Read the model definition and answer for the solid it produces. Units are mm, in the model's axes. Give positions to 0.01 mm unless a question says otherwise; leave off trailing zeros. Write each loop counter-clockwise with the first axis right and the second up, starting at its lowest first coordinate (ties: lowest second). Pieces come first, ordered by that corner, then holes. Notation, with made-up numbers: M -14.5,45.5 L 31.5,45.5 A13 ccw 31.5,52.5 Z; hole C 9.25,55 d4. An arc over 180 degrees is marked long. Put each result on its own line as item: value.
Autodesk Inventor part; units mm, degrees
ref_plane "YZ Plane" through (0, 0, 0) normal (1, 0, 0) x (0, 1, 0)
ref_plane "XZ Plane" through (0, 0, 0) normal (0, 1, 0) x (-1, 0, 0)
ref_plane "XY Plane" through (0, 0, 0) normal (0, 0, 1) x (1, 0, 0)
sketch "スケッチ2" plane through (0, 0, 0) normal (0, 1, 0) x (-1, 0, 0)
  circle A0 centre (366.8992, 83.5559) radius 3
  circle A1 centre (432.0925, 120.7557) radius 3
  arc A2 (460.0993, 143.4366) -> (457.2735, 146.2345) centre (458.5344, 144.682) ccw
  arc A3 (400.439, 89.2207) -> (460.0993, 143.4366) centre (263.302, 300.0629) ccw
  arc A4 (391.277, 83.6402) -> (400.439, 89.2207) centre (301.619, 241.1522) ccw
  arc A5 (372.7132, 76.1699) -> (391.277, 83.6402) centre (354.4726, 148.2986) ccw
  arc A6 (360.1081, 74.8804) -> (372.7132, 76.1699) centre (362.0183, 118.4608) ccw
  arc A7 (355.7086, 75.8282) -> (360.1081, 74.8804) centre (360.696, 88.2936) ccw
  arc A8 (354.3762, 83.2451) -> (355.7086, 75.8282) centre (357.3588, 79.9528) ccw
  arc A9 (361.0987, 88.3442) -> (354.3762, 83.2451) centre (386.9085, 47.3355) ccw
  arc A10 (385.4553, 102.095) -> (361.0987, 88.3442) centre (517.0615, -159.4623) ccw
  arc A11 (385.4553, 102.095) -> (400.8032, 109.8486) centre (-2010.0977, 4863.0707) ccw
  arc A12 (400.8032, 109.8486) -> (428.5996, 125.6368) centre (247.4107, 412.2703) ccw
  arc A13 (428.5996, 125.6368) -> (457.2735, 146.2345) centre (269.2327, 377.7487) ccw
  circle A14 centre (287.1934, 37.1564) radius 3
  circle A15 centre (359.7933, 56.2153) radius 3
  arc A16 (392.7161, 70.8747) -> (390.7107, 74.3087) centre (391.5269, 72.4828) ccw
  arc A17 (321.0565, 33.9474) -> (392.7161, 70.8747) centre (243.1623, 273.099) ccw
  arc A18 (310.7624, 30.9284) -> (321.0565, 33.9474) centre (264.9264, 206.2785) ccw
  arc A19 (290.8977, 28.5173) -> (310.7624, 30.9284) centre (291.9468, 102.9093) ccw
  arc A20 (278.3883, 30.5342) -> (290.8977, 28.5173) centre (291.5128, 72.1352) ccw
  arc A21 (274.384, 32.5883) -> (278.3883, 30.5342) centre (282.4278, 43.3382) ccw
  arc A22 (275.0166, 40.0974) -> (274.384, 32.5883) centre (277.0456, 36.1453) ccw
  arc A23 (282.8299, 43.2828) -> (275.0166, 40.0974) centre (297.1464, -3.0086) ccw
  arc A24 (309.9154, 50.2611) -> (282.8299, 43.2828) centre (369.3413, -236.446) ccw
  arc A25 (309.9154, 50.2611) -> (326.7472, 53.7782) centre (-771.7798, 5269.0252) ccw
  arc A26 (326.7472, 53.7782) -> (357.6827, 61.8342) centre (256.8539, 385.5961) ccw
  arc A27 (357.6827, 61.8342) -> (390.7107, 74.3087) centre (268.9975, 346.6028) ccw
  circle A28 centre (20.0666, -1.5588) radius 5
  circle A29 centre (130.4331, -10.1322) radius 5
  arc A30 (313.248, 18.4984) -> (312.0524, 22.2894) centre (312.4376, 20.3268) ccw
  arc A31 (100.6618, -32.4332) -> (313.248, 18.4984) centre (68.6386, 570.3585) ccw
  arc A32 (74.9225, -33.0376) -> (100.6618, -32.4332) centre (77.5861, 401.9345) ccw
  arc A33 (27.374, -26.2879) -> (74.9225, -33.0376) centre (76.0159, 145.5175) ccw
  arc A34 (-0.3728, -13.8419) -> (27.374, -26.2879) centre (55.8939, 74.446) ccw
  arc A35 (-8.3795, -6.5926) -> (-0.3728, -13.8419) centre (16.9451, 13.3315) ccw
  arc A36 (-2.2486, 10.4222) -> (-8.3795, -6.5926) centre (0, 0) ccw
  arc A37 (17.8428, 12.9532) -> (-2.2486, 10.4222) centre (22.277, -103.2534) ccw
  arc A38 (84.9679, 12.306) -> (17.8428, 12.9532) centre (44.6377, -689.2581) ccw
  arc A39 (84.9679, 12.306) -> (126.1724, 10.004) centre (819.0754, 12782.4716) ccw
  arc A40 (126.1724, 10.004) -> (202.8919, 9.4636) centre (170.258, 822.6468) ccw
  arc A41 (202.8919, 9.4636) -> (312.0524, 22.2894) centre (174.1884, 724.7085) ccw
  line L0 (400.439, 89.2207) -> (374.6007, 72.4148)
  line L1 (374.6007, 72.4148) -> (391.2826, 74.4678)
  line L2 (355.7086, 75.8282) -> (369.1755, 70.4401)
  line L3 (369.1755, 70.4401) -> (326.7472, 53.7782)
  line L4 (321.0565, 33.9474) -> (289.8884, 23.7957)
  line L5 (289.8884, 23.7957) -> (312.5672, 22.3226)
  line L6 (278.3883, 30.5342) -> (291.6044, 26.3646)
  line L7 (291.6044, 26.3646) -> (243.2783, 12.2299)
  point P0 (0, 0)
extrude "押し出し2" add sketch "スケッチ2" along normal blind 4
fillet "フィレット2" radius 3 4 edges at (-369.1755, 2, 70.4401) (-291.6044, 2, 26.3646) (-374.6007, 2, 72.4148) (-289.8884, 2, 23.7957)
fillet "フィレット2" radius 100 2 edges at (-326.7472, 2, 53.7782) (-243.2783, 2, 12.2299)
sketch "スケッチ3" plane through (0, 0, 0) normal (0, -1, 0) x (1, 0, 0)
  circle A0 centre (-20.0666, -1.5588) radius 6
  circle A1 centre (-130.4331, -10.1322) radius 6
  circle A2 centre (-130.4331, -10.1322) radius 5
  circle A3 centre (-20.0666, -1.5588) radius 5
  point P0 (0, 0)
  dimension "d10" = 12
  dimension "d11" = 12
extrude "押し出し3" cut sketch "スケッチ3" against normal through all
equation "\"d11\" = d10"
properties part number "bracket2" material "木材 (オーク)"
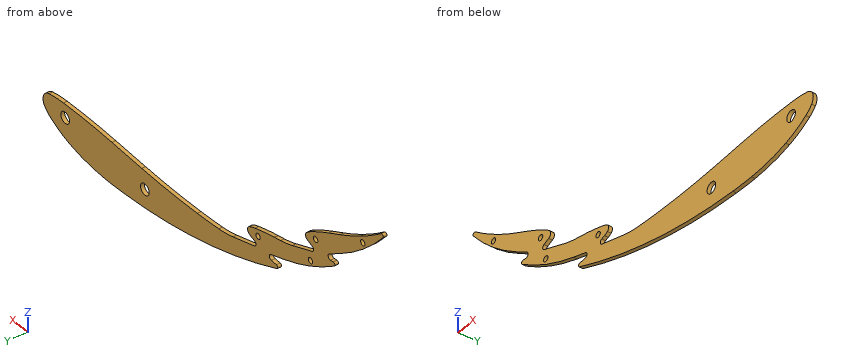
(1) Section A-A on y = 1.3 is taken. Give the number of separate pieces and of enclosed holes in the cut face, and give its area (3 significant figures).
Result:
separate pieces: 1
enclosed holes: 6
area: 13,600 mm²
(2) Given pin 1 Ø1.5 at (y, z) = (3.5, 93.5) entering from -X; pin 2 Ø1 at (x, y) = (-281, 3) entering from -Z, each flat-ended and moving along its own axis, determine where each tip first touches the part or whether it passes through.
Result:
pin 1: stops at x = -407.88
pin 2: stops at z = 5.12
(3) Straight lines are drawn through the part: line 1 along Z through (x, y) = (-387, 1.8); line 2 along Z through (x, y) = (-84, 0.7); line 3 along Z through (x, y) = (-431.5, 0.3). For each, find the intervals that lie inside material, in ascending order. Write a range as from..to.
Result:
line 1: z = 66.77..73.98, 80.48..102.87
line 2: z = -33..12.36
line 3: z = 113.06..117.81, 123.7..127.49
(4) Section B-B on x = -165 is taken. Determine the outline of the cut face in (y, z), and give its area (3 significant figures).
Result:
outline: M 0,-25.54 L 4,-25.54 L 4,8.83 L 0,8.83 Z
area: 137 mm²
(5) Section C-C on z = -21.5 is taken. Determine the outline of the cut face in (x, y), and give its area (3 significant figures).
Result:
outline: M -187.33,0 L -14,0 L -14,4 L -187.33,4 Z
area: 693 mm²
